The listing builds one solid part. Answer for the finished solid, in the listing's coordinates (mm). A direction names the side the tool comes from. Give positions to 0.01 mm unless a question says otherwise; leave off trailing zeros. Order: outer loops, then holes, each group sorted by start corner. A loop starts at its lowest first (then second) coordinate and runs counter-clockwise, first axis right, second up. Notation, with made-up numbers: (42.25, -20.75) - (84.25, -20.75) arc R18 ccw to (84.25, 11.25) - close; hole circle Ø6 at (43.5, -3.5). An arc over 180 degrees is marked (long way). Answer as a JSON object with one key per item and string values. Group by question number.
Q1. The mould has two halves that part along Z. Classify faces 1 (the face through (13, -1, -1)), 2 (the face through (11.479, -3.905, 0.867)), 3 (the face through (10, 0, 0)), 4 (the face through (12.01, -0.95, 0.02)): released by +Z, released by -Z, zero draft, split by the parting line, or undercut.
Q2. A cutting plane is placed at A-A, the plane x = 3. Give the vertices of the cut face in (y, z).
Q3. Consider line 1 (Y direction, x = 4.5, z = 0); line 2 (Z direction, x = 8.5, y = 0); line 3 (Z direction, x = 9.5, y = -1). Determine where each line is inside the solid, lowest interval first.
Q4. For faces 5 (the face through (0, -2, -1)), 6 (the face through (12, 1, -0.95)), 7 (the face through (12.65, 2.99, -0.64)), 8 (the face through (5, 1.5, 0)), determine the directions among +Z, -Z, +X, -X, +Y, -Y from which every point of the face is accessible in a straight line to the end or side of a thin tool.
Q5. Given pin 1 (2 mm diameter, centred on x = 11.5, y = 1.5, fed in from -Z); pin 2 (1 mm diameter, centred on x = 11.5, y = 1, fed in from +Z); pin 3 (0.5 mm diameter, centred on x = 12.5, z = 0.5, fed in from -Y), each flat-ended and moving along its own axis, determine where each tip first touches the part or whether it passes through.
from build123d import *

# Parameters (mm, degrees)
SKETCH2_R           = 3
BOSS_EXTRUDE1_DEPTH = 10
SKETCH3_R           = 4
BOSS_EXTRUDE2_DEPTH = 3
FILLET1_R           = 2
CUT_EXTRUDE1_DEPTH  = 2
SKETCH6_R           = 0.95
CUT_EXTRUDE2_DEPTH  = 15.866068747


with BuildPart() as part:
    # Sketch2 → Boss-Extrude1 (new body)
    with BuildSketch(Plane(origin=(0, 0, 0), x_dir=(0, 0, -1), z_dir=(1, 0, 0))):
        Circle(SKETCH2_R)
        with BuildLine():
            Line((-1.322875656, 1.5), (1.322875656, 1.5))
            ThreePointArc((1.322875656, 1.5), (0, -2), (-1.322875656, 1.5))
        make_face(mode=Mode.SUBTRACT)
    extrude(amount=BOSS_EXTRUDE1_DEPTH)

    # Sketch3 → Boss-Extrude2 (add)
    with BuildSketch(Plane(origin=(10, 0, 0), x_dir=(0, 0, -1), z_dir=(1, 0, 0))):
        Circle(SKETCH3_R)
    extrude(amount=BOSS_EXTRUDE2_DEPTH)

    # Fillet1
    # the kernel refuses this fillet: 2 mm, written as the material it adds along each edge
    with BuildSketch(Plane(origin=(10, 0, 0), x_dir=(0, 0, -1), z_dir=(0, -1, 0))) as fillet1_piece_1:
        with BuildLine():
            CenterArc((5, -1.732050808), FILLET1_R, 120, 60)
            Line((3, -1.732050808), (2.96, -1.732050808))
            Line((2.96, -1.732050808), (2.96, 0))
            Line((2.96, 0), (3, 0.04))
            ThreePointArc((3, 0.04), (3.5, 0.04), (3.98, 0.034641016))
            Line((3.98, 0.034641016), (4, 0))
        make_face()
    revolve(axis=Axis((10, 0, 0), (1, 0, 0)))

    # Sketch4 → Cut-Extrude1 (cut)
    with BuildSketch(Plane(origin=(13, 0, 0), x_dir=(0, 0, -1), z_dir=(1, 0, 0))):
        with BuildLine():
            Line((-0.95, 2), (-0.95, 0))
            ThreePointArc((-0.95, 0), (0, -0.95), (0.95, 0))
            Line((0.95, 0), (0.95, 2))
            Line((0.95, 2), (-0.95, 2))
        make_face()
    extrude(amount=-CUT_EXTRUDE1_DEPTH, mode=Mode.SUBTRACT)

    # Sketch6 → Cut-Extrude2 (cut, through all)
    with BuildSketch(Plane(origin=(0, 2, 0), x_dir=(-1, 0, 0), z_dir=(0, -1, 0))):
        with Locations((-11.95, 0)):
            Circle(SKETCH6_R)
    extrude(amount=-CUT_EXTRUDE2_DEPTH, mode=Mode.SUBTRACT)


solid = part.part
Reply:
{
 "1": {"face 1": "zero draft", "face 2": "split by the parting line", "face 3": "undercut", "face 4": "undercut"},
 "2": {"outline": "circle Ø6 at (0, 0); hole (1.5, -1.32) - (1.5, 1.32) arc R2 ccw (long way) to start"},
 "3": {"line 1": "y = -3 to -2, 1.5 to 3", "line 2": "z = -3.01 to -2, 2 to 3.01", "line 3": "z = -3.28 to -1.73, 1.73 to 3.28"},
 "4": {"face 5": "+Z, -Z, -X, +Y, -Y", "face 6": "+X", "face 7": "+Y", "face 8": "-X"},
 "5": {"pin 1": "stops at z = -3.97", "pin 2": "stops at z = 3.97", "pin 3": "stops at y = -3.99"}
}
